from build123d import *

# Parameters (mm, degrees)
SKETCH2_W               = 0.4
SKETCH2_H               = 3.255003129
EXTRUDED_CUT1_DEPTH     = 17
EXTRUDED_CUT2_DEPTH     = 17
CIRCULAR_PATTERN1_COUNT = 8


with BuildPart() as part:
    # Sketch1 → Rotation1 (revolve)
    with BuildSketch(Plane.XY, mode=Mode.PRIVATE) as rotation1_sk:
        Polygon((-4, -4.5), (-4, 13.5), (-5.102698732, 13.5), (-7, 0), (-6, 0), (-6, -2), (-7.25, -2), (-5.806624327, -4.5), align=None)
    revolve(rotation1_sk.sketch.rotate(Axis((0, 0, 0), (0, 1, 0)), 270), axis=Axis((0, 0, 0), (0, 1, 0)))

    # Sketch2 → Extruded Cut1 (cut)
    with BuildSketch(Plane.XZ.offset(4.5)):
        with Locations((0, 5.622498436)):
            Rectangle(SKETCH2_W, SKETCH2_H)
    extruded_cut1 = extrude(amount=-EXTRUDED_CUT1_DEPTH, mode=Mode.SUBTRACT)

    # Sketch3 → Extruded Cut2 (cut)
    with BuildSketch(Plane(origin=(0, 13.5, 0), x_dir=(1, 0, 0), z_dir=(0, 1, 0))):
        Polygon((-0.185436771, -0.074921319), (-2.901334573, 6.647161627), (-2.530461031, 6.797004264), (0.185436771, 0.074921319), align=None)
    extruded_cut2 = extrude(amount=-EXTRUDED_CUT2_DEPTH, mode=Mode.SUBTRACT)

    # Circular Pattern1: Extruded Cut1, Extruded Cut2 ×8 about axis
    circular_pattern1_axis = Axis((0, 0, 0), (0, 1, 0))
    add([extruded_cut1.rotate(circular_pattern1_axis, i * 360 / CIRCULAR_PATTERN1_COUNT) for i in range(1, CIRCULAR_PATTERN1_COUNT)], mode=Mode.SUBTRACT)
    add([extruded_cut2.rotate(circular_pattern1_axis, i * 360 / CIRCULAR_PATTERN1_COUNT) for i in range(1, CIRCULAR_PATTERN1_COUNT)], mode=Mode.SUBTRACT)


solid = part.part
For this review, take the finished solid that the model builds, in its own axes (mm). A direction names the side the tool comes from. Round coordinates to 2 decimals unless told otherwise and drop trailing zeros. Write item = value, one per line. Start each with the question number.
1. For pin 1 Ø1 at (y, z) = (7, -3) entering from -X; pin 2 Ø1.5 at (x, y) = (-5.5, 1) entering from +Z; pin 3 Ø0.7 at (x, z) = (-1.5, 6.5) entering from -Y; pin 4 Ø1.6 at (x, z) = (-4, -5) entering from -Y, all flat-tipped, find the tip position at first contact; note any pin that passes through.
2. For faces 5 (the face through (-5, 0, 4)), 6 (the face through (3, 12.5, 3)), 7 (the face through (5.877, -1.014, 1.21)), 8 (the face through (4.973, 3.23, -1.793)), 9 (the face through (-4.967, -1.014, -3.366)), list the 3-axis set-ups (+Z, -Z, +X, -X, +Y, -Y) from which the entire face can be reached by the end or side of a thin tool; tool diameter is ignored.
3. Wall thickness on L1, parallel to X at y = 4, z = -5.5; L2, parallel to Z at x = -5.25, y = 4; L3, parallel to X at y = 2.5, z = 3.5: over which ranges is each line inside the solid? List them lowest first.
4. Draft analysis for pull direction Z (two halves, no side actions). For faces 1 (the face through (-4.675, 6.655, 3.863)), 2 (the face through (-6.05, 6.66, 0.41)), 3 (the face through (4, -2, 5)), 4 (the face through (3, 12.5, -3)), state which applies: released by +Z, released by -Z, zero draft, split by the parting line, or undercut.
5. Consider section A-A on y = -0.75. Give the number of separate pieces and of enclosed holes in the cut face, plus the area to 3 significant figures.
Evaluation:
q1.pin_1 = -5.48
q1.pin_2 = 4.77
q1.pin_3 = -3.61
q1.pin_4 = -4.5
q2.face_5 = +Z, -X
q2.face_6 = -Y
q2.face_7 = +Z, +X
q2.face_8 = +Y
q2.face_9 = -Z, -X
q3.L1 = -3.35 to -2.44, -2.01 to -0.2, 0.2 to 2.12, 2.55 to 3.35
q3.L2 = -3.73 to -2.45, -2.01 to -0.2, 0.2 to 1.91, 2.34 to 3.73
q3.L3 = -5.65 to -3.78, -3.22 to -1.94, 1.94 to 3.22, 3.78 to 5.65
q4.face_1 = released by +Z
q4.face_2 = split by the parting line
q4.face_3 = zero draft
q4.face_4 = undercut
q5.separate_pieces = 16
q5.enclosed_holes = 0
q5.area = 50.0 mm2
